```python
from build123d import *

# Parameters (mm, degrees)
EXTRUDE_1_DEPTH     = 234.733197
SKETCH_2_R          = 5
CUT_EXTRUDE_1_DEPTH = 31


with BuildPart() as part:
    # Эскиз1 → Бобышка-Вытянуть1 (new body)
    with BuildSketch(Plane.XY):
        with BuildLine():
            Line((-12, 0), (12, 0))
            ThreePointArc((12, 0), (14.121320344, -0.878679656), (15, -3))
            Line((15, -3), (15, -27))
            ThreePointArc((15, -27), (14.121320344, -29.121320344), (12, -30))
            Line((12, -30), (-12, -30))
            ThreePointArc((-12, -30), (-14.121320344, -29.121320344), (-15, -27))
            Line((-15, -27), (-15, -3))
            ThreePointArc((-15, -3), (-14.121320344, -0.878679656), (-12, 0))
        make_face()
        with BuildLine():
            Line((-11, -2), (11, -2))
            ThreePointArc((11, -2), (12.414213562, -2.585786438), (13, -4))
            Line((13, -4), (13, -26))
            ThreePointArc((13, -26), (12.414213562, -27.414213562), (11, -28))
            Line((11, -28), (-11, -28))
            ThreePointArc((-11, -28), (-12.414213562, -27.414213562), (-13, -26))
            Line((-13, -26), (-13, -4))
            ThreePointArc((-13, -4), (-12.414213562, -2.585786438), (-11, -2))
        make_face(mode=Mode.SUBTRACT)
    extrude(amount=-EXTRUDE_1_DEPTH)

    # Эскиз2 → Вырез-Вытянуть1 (cut, through all)
    with BuildSketch(Plane(origin=(0, 0, 0), x_dir=(1, 0, 0), z_dir=(0, 1, 0))):
        with Locations((2.5, 57)):
            Circle(SKETCH_2_R)
    extrude(amount=-CUT_EXTRUDE_1_DEPTH, mode=Mode.SUBTRACT)


solid = part.part
```
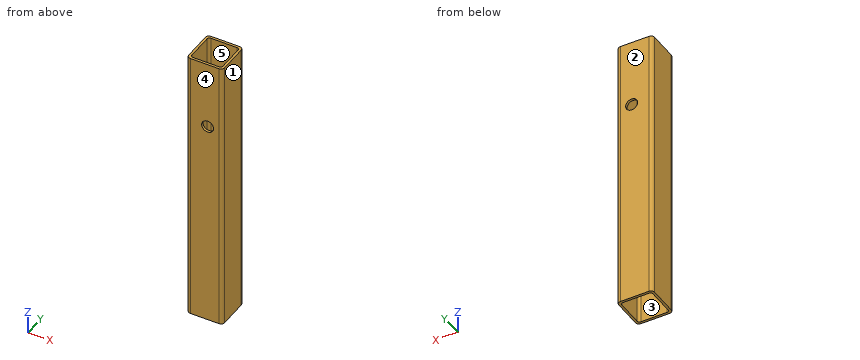
Read the model definition and answer for the solid it produces. Units are mm, in the model's axes. Face numbers are marked on the shaded views. A direction names the side the tool comes from. Give positions to 0.01 mm unless a question says otherwise; leave off trailing zeros. Order: outer loops, then holes, each group sorted by start corner. A loop starts at its lowest first (then second) coordinate and runs counter-clockwise, first axis right, second up. Notation, with made-up numbers: (64.25, 49.5) -> (94.25, 49.5) arc R27 ccw to (94.25, 68.5) -> close; hole circle Ø4 at (51.25, 11.25). An arc over 180 degrees is marked (long way). One line per item, written item: value. Start each with the question number.
(1) The part is cut by section D-D (z = -57). Determine the outline of the cut face in (x, y).
(2) The part is cut by section C-C (x = 2.5). Determine the outline of the cut face in (y, z), and give its area (3 significant figures).
(3) A flat-ended cylindrical pin translates along its axis: P1, Ø8, axis at x = 2.5, z = -57, coming from the +Y side. Find the tip coordinate at first contact, or state that the pin passes through.
(4) For a pull along Y with two mould halves and no side action, classify the marked faces 1, 2 and 3 as released by +Y, released by -Y, zero draft, split by the parting line, or undercut.
(5) A tool of negligible diameter and unlimited length cuts with its end or side. For the marked faces 4 and 5, from which of +Z, -Z, +X, -X, +Y, -Y can it reach the whole face along a straight path? Write none if from no direction.
(6) The part is cut by section A-A (z = -129). Determine the outline of the cut face in (x, y), and give its area (3 significant figures).
(7) Straight lines are drawn through the part: L1, parallel to X at y = -22.25, z = -110; L2, parallel to Y at x = 8.5, z = -72.5; L3, parallel to Z at x = 2.5, y = -28.8. For each, find the intervals that lie inside material, in ascending order.
(8) The part is cut by section B-B (y = -8.25). Determine the outline of the cut face in (x, z).
Taken from the geometry:
1. outline: (-15, -27) arc R3 ccw to (-12, -30) -> (-2.5, -30) -> (-2.5, -28) -> (-11, -28) arc R2 cw to (-13, -26) -> (-13, -4) arc R2 cw to (-11, -2) -> (-2.5, -2) -> (-2.5, 0) -> (-12, 0) arc R3 ccw to (-15, -3) -> close; (7.5, -30) -> (12, -30) arc R3 ccw to (15, -27) -> (15, -3) arc R3 ccw to (12, 0) -> (7.5, 0) -> (7.5, -2) -> (11, -2) arc R2 cw to (13, -4) -> (13, -26) arc R2 cw to (11, -28) -> (7.5, -28) -> close
2. outline: (-30, -234.73) -> (-28, -234.73) -> (-28, -62) -> (-30, -62) -> close; (-30, -52) -> (-28, -52) -> (-28, 0) -> (-30, 0) -> close; (-2, -234.73) -> (0, -234.73) -> (0, -62) -> (-2, -62) -> close; (-2, -52) -> (0, -52) -> (0, 0) -> (-2, 0) -> close
2. area: 899 mm^2
3. P1: through
4. face 1: zero draft
4. face 2: released by +Y
4. face 3: undercut
5. face 4: +Z, -Z, +X, -X, -Y
5. face 5: +Z, -Z
6. outline: (-15, -27) arc R3 ccw to (-12, -30) -> (12, -30) arc R3 ccw to (15, -27) -> (15, -3) arc R3 ccw to (12, 0) -> (-12, 0) arc R3 ccw to (-15, -3) -> close; hole (-13, -26) arc R2 ccw to (-11, -28) -> (11, -28) arc R2 ccw to (13, -26) -> (13, -4) arc R2 ccw to (11, -2) -> (-11, -2) arc R2 ccw to (-13, -4) -> close
6. area: 220 mm^2
7. L1: -15 to -13, 13 to 15
7. L2: -30 to -28, -2 to 0
7. L3: -234.73 to -62, -52 to 0
8. outline: (-15, -234.73) -> (-13, -234.73) -> (-13, 0) -> (-15, 0) -> close; (13, -234.73) -> (15, -234.73) -> (15, 0) -> (13, 0) -> close
